Build history of the part. All positions in model axes, mm. A direction names the side the tool comes from. Round coordinates to 2 decimals unless told otherwise and drop trailing zeros. Write each loop counter-clockwise with the first axis right and the second up, starting at its lowest first coordinate (ties: lowest second). Pieces come first, ordered by that corner, then holes.
Item 1: Band-saw the part on B-B, the plane y = -35.5. Write the cut outline in (x, z).
Item 2: Band-saw the part on C-C, the plane x = 190. Write the cut outline in (y, z), then the cut area to 3 significant figures.
Item 3: Band-saw the part on D-D, the plane y = 57.5. Write the cut outline in (x, z).
Item 4: Band-saw the part on A-A, the plane z = -106. Write the cut outline in (x, y).
Item 5: Wall check: probe 1 along Y at (x, z) = (65.35, -130); probe 2 along Y at (x, z) = (222.65, -130.3); probe 3 along Y at (x, z) = (109, -110). Give the ranges that are in metal, low to high.
Item 6: 3-axis set-ups, long thin cutter, end or side, ignore diameter. For faces 1 (the flat face through (156, -44, -112)), 2 (the flat face through (212, -5, -112)), 3 (the flat face through (156, 36, -112)): which of +Z, -Z, +X, -X, +Y, -Y reach the whole face in a straight line?
Item 7: Drop flat-ended pins along their axis: pin 1 Ø24 at (x, y) = (153, 10) entering from +Z; pin 2 Ø10.5 at (x, z) = (176, -116.5) entering from -Y; pin 3 Ø1.3 at (y, z) = (-14.5, -130) entering from +X; pin 4 Ø6 at (y, z) = (-60.5, -124) entering from +X. Give the stop position or say it passes through.
Item 8: Mould opens along X. For faces 4 (the flat face through (151, 70, -86)), 5 (the flat face through (222.217, 58.532, -110.65)), 6 (the cylindrical face through (223.573, 49.206, -130.211)) say: +X half, -X half, draft (parallel to the pull), parting line (faces both ways), or undercut.
```python
from build123d import *

# Parameters (mm, degrees)
SKETCH004_W  = 170
SKETCH004_H  = 170
SKETCH004_R  = 2
PAD004_DEPTH = 1.6
PAD007_DEPTH = 45
SKETCH042_W  = 110
SKETCH042_H  = 80
PAD022_DEPTH = 36
PAD029_DEPTH = 5


with BuildPart() as part:
    # Sketch004 → Pad004 (new body)
    with BuildSketch(Plane.XY):
        with Locations((85, 85)):
            Rectangle(SKETCH004_W, SKETCH004_H)
        with Locations((6.35, 4.8997)):
            Circle(SKETCH004_R, mode=Mode.SUBTRACT)
        with Locations((163.65, 4.8997)):
            Circle(SKETCH004_R, mode=Mode.SUBTRACT)
        with Locations((6.35, 159.84)):
            Circle(SKETCH004_R, mode=Mode.SUBTRACT)
        with Locations((163.65, 136.98)):
            Circle(SKETCH004_R, mode=Mode.SUBTRACT)
    extrude(amount=PAD004_DEPTH)

    # Sketch010 → Pad007 (join)
    with BuildSketch(Plane.XY):
        Polygon((12, 174), (12, 138), (151.758911, 138), (175, 151.249695), (175, 174), align=None)
    extrude(amount=PAD007_DEPTH)

    # Sketch042 → Pad022 (join)
    with BuildSketch(Plane.XY):
        with Locations((98, 82)):
            Rectangle(SKETCH042_W, SKETCH042_H)
    extrude(amount=PAD022_DEPTH)

    # Sketch010 → Pad029 (join)
    with BuildSketch(Plane.XY):
        Polygon((12, 174), (12, 138), (151.758911, 138), (175, 151.249695), (175, 174), align=None)
    extrude(amount=-PAD029_DEPTH)


with BuildPart() as part_1:
    # Body002 placement: moved
    add(part.part.moved(Location((59, -86, -131))))


solid = part_1.part
```
Results:
1. outline: (59, -131) - (229, -131) - (229, -129.4) - (212, -129.4) - (212, -95) - (102, -95) - (102, -129.4) - (59, -129.4) - close
2. outline: (-86, -131) - (52, -131) - (52, -136) - (88, -136) - (88, -86) - (52, -86) - (52, -129.4) - (36, -129.4) - (36, -95) - (-44, -95) - (-44, -129.4) - (-86, -129.4) - close
2. area: 4,770 mm2
3. outline: (59, -131) - (71, -131) - (71, -136) - (220.41, -136) - (220.41, -131) - (229, -131) - (229, -129.4) - (220.41, -129.4) - (220.41, -86) - (71, -86) - (71, -129.4) - (59, -129.4) - close
4. outline: (71, 52) - (210.76, 52) - (234, 65.25) - (234, 88) - (71, 88) - close; (102, -44) - (212, -44) - (212, 36) - (102, 36) - close
5. probe 1: y = -86 to -83.1, -79.1 to 71.84, 75.84 to 84
5. probe 2: y = -86 to -83.1, -79.1 to 48.98, 52.98 to 88
5. probe 3: y = -44 to 36, 52 to 88
6. face 1: +Z, +X, -X, -Y
6. face 2: +Z, +X, -Y
6. face 3: +Z, +X, -X
7. pin 1: stops at z = -95
7. pin 2: stops at y = -44
7. pin 3: stops at x = 229
7. pin 4: passes through
8. face 4: draft
8. face 5: +X half
8. face 6: undercut
